```python
from build123d import *

# Parameters (mm, degrees)
SKETCH1_R           = 0.75
BOSS_EXTRUDE1_DEPTH = 4
SKETCH2_R           = 1.5
BOSS_EXTRUDE2_DEPTH = 4.2


with BuildPart() as part:
    # Sketch1 → Boss-Extrude1 (new body)
    with BuildSketch(Plane(origin=(0, 0, 0), x_dir=(0, 0, -1), z_dir=(1, 0, 0))):
        with BuildLine():
            Line((71.658914309, 8.5), (24.158914309, 8.5))
            ThreePointArc((24.158914309, 8.5), (8.750910997, 12.358734302), (-1.484840821, 0.212715152))
            ThreePointArc((-1.484840821, 0.212715152), (-0.212715152, -1.484840821), (1.484840821, -0.212715152))
            ThreePointArc((1.484840821, -0.212715152), (10.256916266, 9.676453105), (22.798933484, 5.5))
            Line((22.798933484, 5.5), (71.658914309, 5.5))
            ThreePointArc((71.658914309, 5.5), (73.158914309, 7), (71.658914309, 8.5))
        make_face()
        with Locations((71.658914309, 7)):
            Circle(SKETCH1_R, mode=Mode.SUBTRACT)
    extrude(amount=BOSS_EXTRUDE1_DEPTH)

    # Sketch2 → Boss-Extrude2 (add)
    with BuildSketch(Plane(origin=(4, 0, 0), x_dir=(0, 0, -1), z_dir=(1, 0, 0))):
        with Locations(Location((0, 0, 0), (0, 0, 171.847397423))):
            Circle(SKETCH2_R)
    extrude(amount=BOSS_EXTRUDE2_DEPTH)


solid = part.part
```
Design review of the part built by this model. Coordinates are the model's own, in mm. A direction names the side the tool comes from. Round coordinates to 2 decimals unless told otherwise and drop trailing zeros. Order: outer loops, then holes, each group sorted by start corner. A loop starts at its lowest first (then second) coordinate and runs counter-clockwise, first axis right, second up. Notation, with made-up numbers: (38, -19.5) - (94, -19.5) arc R8 ccw to (94, -12.5) - close; hole circle Ø6 at (50.5, 6). An arc over 180 degrees is marked (long way). One line per question, with ' | ' between items.
Item 1: Take a section at B-B, the plane y = 7. Write out the cut boundary in (x, z).
Checks:
outline: (0, -73.16) - (4, -73.16) - (4, -72.41) - (0, -72.41) - close; (0, -70.91) - (4, -70.91) - (4, -21.4) - (0, -21.4) - close; (0, -5.33) - (4, -5.33) - (4, -1.3) - (0, -1.3) - close
Item 2: Wall thickness on line 1 (Y direction, x = 1.25, z = -35.5); line 2 (Z direction, x = 7.5, y = -0.25); line 3 (X direction, y = 8.5, z = -21): over which ranges is each line inside the solid? List them lowest first. Write a range as [from, to].
Checks:
line 1: [5.5, 8.5] | line 2: [-1.48, 1.48] | line 3: [0, 4]
Item 3: Draft analysis for pull direction Z (two halves, no side actions). For faces 1 (the face through (1.972, 12.429, -8.974)), 2 (the face through (1.97, 7.03, -70.91)), 3 (the face through (2, 5.5, -47)), state which applies: +Z half, -Z half, draft (parallel to the pull), parting line (faces both ways), or undercut.
Checks:
face 1: parting line | face 2: undercut | face 3: draft
Item 4: Take a section at A-A, the plane x = 1. Write out the cut boundary in (y, z), then the cut area to 3 significant figures.
Checks:
outline: (-0.21, -1.48) arc R12 cw to (5.5, -22.8) - (5.5, -71.66) arc R1.5 ccw to (8.5, -71.66) - (8.5, -24.16) arc R15 ccw to (0.21, 1.48) arc R1.5 ccw to start; hole circle Ø1.5 at (7, -71.66) | area: 242 mm²
Item 5: Machinability: for faces 4 (the face through (0, 7, -30)), 5 (the face through (2, 8.5, -48)), which of the approach directions +Z, -Z, +X, -X, +Y, -Y give a long, thin tool a straight path to every point of the face, cutting with its end or side? Answer none if there is none.
Checks:
face 4: +Z, -Z, -X, +Y, -Y | face 5: -Z, +X, -X, +Y
Item 6: Take a section at D-D, the plane x = 6. Write out the cut boundary in (y, z), then the cut area to 3 significant figures.
Checks:
outline: circle Ø3 at (0, 0) | area: 7.07 mm²
Item 7: Take a section at C-C, the plane z = 0. Write out the cut boundary in (x, y), then the cut area to 3 significant figures.
Checks:
outline: (0, -1.5) - (8.2, -1.5) - (8.2, 1.5) - (4, 1.5) - (4, 4.9) - (0, 4.9) - close | area: 38.2 mm²
Item 8: For P1, Ø3, axis at y = 4.5, z = -26.5, coming from the +X side; P2, Ø1, axis at x = 3, y = 8, coming from the +Z side; P3, Ø3, axis at x = 4.5, y = 11, coming from the +Z side; P4, Ø2, axis at y = 7, z = -71.66, coming from the -X side, all flat-tipped, find the tip position at first contact; note any pin that passes through.
Checks:
P1: x = 4 | P2: z = -1.69 | P3: z = -3.73 | P4: x = 0
